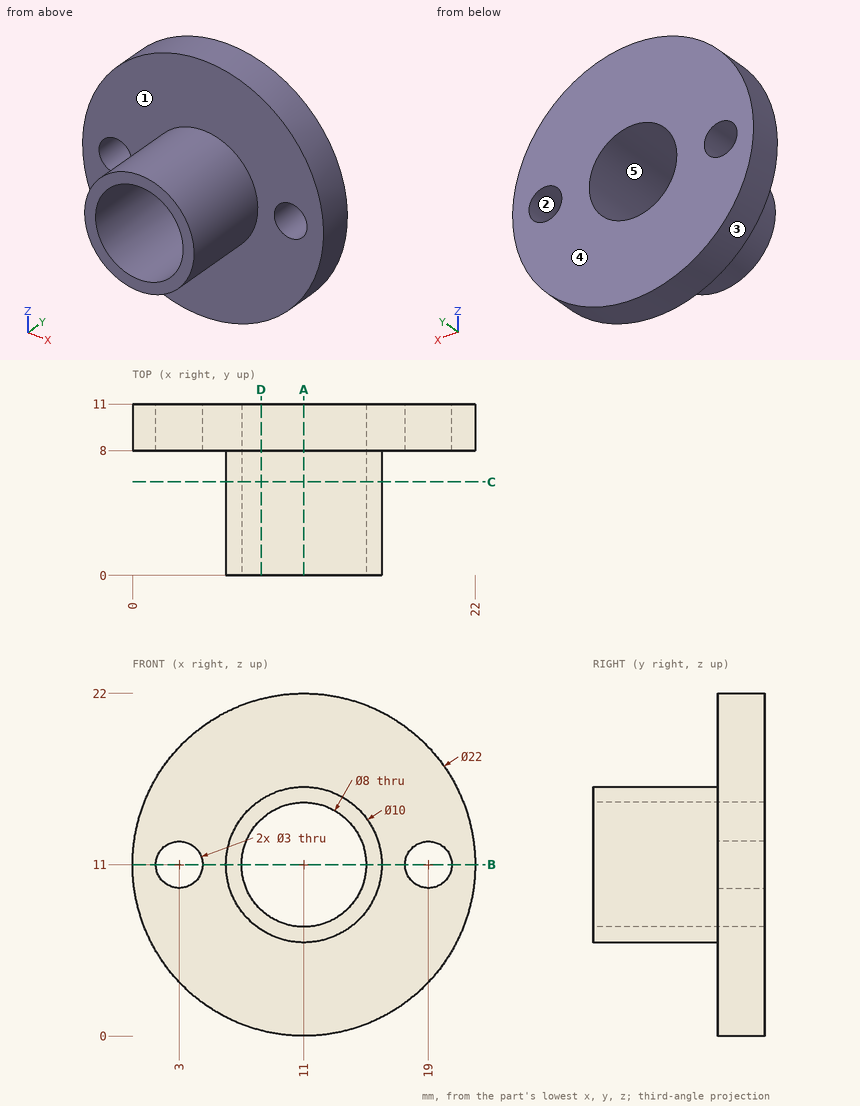
For this review, use the dimensioned drawing (mm, ordinates from the lowest corner) and the shaded views. A direction names the side the tool comes from. Coordinates: 2 decimals unless noted, no trailing zeros. Loops run counter-clockwise (first coordinate to the right, second up) from the corner with the lowest first, then second, coordinate; pieces in that order, holes last. Notation, with made-up numbers: M 17,27.25 L 45,27.25 A16 cw 45,50.25 Z; hole C -40,-26 d4. An arc over 180 degrees is marked long. Answer as CSV lines item,"result".
Item 1: For probe 1 along X at (y, z) = (8.9, 11); probe 2 along Y at (x, z) = (16, 12.25); probe 3 along Z at (x, y) = (13, 1.75), list the stretches that pass through material, from the lowest coordinate up.
Answer list:
probe 1,"0 to 1.5, 4.5 to 7, 15 to 17.5, 20.5 to 22"
probe 2,"8 to 11"
probe 3,"6.42 to 7.54, 14.46 to 15.58"
Item 2: Add section A-A on x = 11. State the section outline as (y, z) points, plus the area to 3 significant figures.
Answer list:
outline,"M 0,6 L 8,6 L 8,0 L 11,0 L 11,7 L 0,7 Z; M 0,15 L 11,15 L 11,22 L 8,22 L 8,16 L 0,16 Z"
area,"58.0 mm²"
Item 3: For P1, Ø2, axis at x = 16.5, y = 5.5, coming from the -Z side; P2, Ø5, axis at x = 18, y = 7.5, coming from the +Z side; P3, Ø2.5, axis at x = 3, z = 11, coming from the +Y side; P4, Ø1, axis at x = 7.5, y = 5, coming from the -Z side, all flat-tipped, find the tip position at first contact; note any pin that passes through.
Answer list:
P1,"z = 8.82"
P2,"z = 21.01"
P3,"through"
P4,"z = 7"
Item 4: Machinability: for the marked faces 1 and 2, which of the approach directions +Z, -Z, +X, -X, +Y, -Y give a long, thin tool a straight path to every point of the face, cutting with its end or side? Answer none if there is none.
Answer list:
face 1,"-Y"
face 2,"+Y, -Y"
Item 5: Add section C-C on y = 6. State the section outline as (x, z) points.
Answer list:
outline,"C 11,11 d10; hole C 11,11 d8"
Item 6: Add section D-D on x = 8.25. State the section outline as (y, z) points, plus the area to 3 significant figures.
Answer list:
outline,"M 0,6.82 L 8,6.82 L 8,0.35 L 11,0.35 L 11,8.1 L 0,8.1 Z; M 0,13.9 L 11,13.9 L 11,21.65 L 8,21.65 L 8,15.18 L 0,15.18 Z"
area,"66.8 mm²"
Item 7: Add section B-B on z = 11. State the section outline as (x, y) points.
Answer list:
outline,"M 0,8 L 1.5,8 L 1.5,11 L 0,11 Z; M 4.5,8 L 6,8 L 6,0 L 7,0 L 7,11 L 4.5,11 Z; M 15,0 L 16,0 L 16,8 L 17.5,8 L 17.5,11 L 15,11 Z; M 20.5,8 L 22,8 L 22,11 L 20.5,11 Z"
Item 8: The part is to be moulded in two halves that separate along X. For the marked faces 3, 4 and 5, say which applies: pulls with the +X half, pulls with the -X half, needs draft (parallel to the pull), parting line crosses it, or undercut.
Answer list:
face 3,"parting line crosses it"
face 4,"needs draft"
face 5,"undercut"
